Geometry: final body of the model. Coordinates: model frame, mm. A direction names the side the tool comes from. Round coordinates to 2 decimals unless told otherwise and drop trailing zeros. Loops run counter-clockwise (first coordinate to the right, second up) from the corner with the lowest first, then second, coordinate; pieces in that order, holes last. Notation, with made-up numbers: (43, 35.5) - (69, 35.5) arc R24 cw to (69, 51.5) - close; hole circle Ø8 at (-17, 15.5). An arc over 180 degrees is marked (long way). Use CSV: the item, a comma, the result in double quotes.
from build123d import *

# Parameters (mm, degrees)
BASE_FLANGE1_DEPTH = 406.4
SKETCH6_R          = 3.175
CUT_EXTRUDE1_DEPTH = 6.35
SKETCH7_R          = 3.429
CUT_EXTRUDE2_DEPTH = 6.35


# Read off the part's stored shape, not the designer's step: Base-Flange1
with BuildPart() as part:
    # Base-Flange1 outline → Base-Flange1 (new body)
    with BuildSketch(Plane(origin=(0, 0, 0), x_dir=(0, 0, -1), z_dir=(1, 0, 0))):
        with BuildLine():
            Line((0, -3.175), (38.1, -3.175))
            Line((38.1, -3.175), (38.1, 0))
            Line((38.1, 0), (0, 0))
            Line((0, 0), (0, 38.1))
            Line((0, 38.1), (-3.175, 38.1))
            Line((-3.175, 38.1), (-3.175, 0))
            ThreePointArc((-3.175, 0), (-2.24506403, -2.24506403), (0, -3.175))
        make_face()
    extrude(amount=BASE_FLANGE1_DEPTH)

    # Sketch6 → Cut-Extrude1 (cut)
    with BuildSketch(Plane.XY.offset(3.175)):
        with Locations((31.75, 19.05)):
            Circle(SKETCH6_R)
        with Locations((374.65, 19.05)):
            Circle(SKETCH6_R)
    extrude(amount=-CUT_EXTRUDE1_DEPTH, mode=Mode.SUBTRACT)

    # Sketch7 → Cut-Extrude2 (cut)
    with BuildSketch(Plane.XZ.offset(3.175)):
        with Locations(Location((25.4, -25.4, 0), (0, 0, 270))):
            Circle(SKETCH7_R)
        with Locations(Location((381, -25.4, 0), (0, 0, 270))):
            Circle(SKETCH7_R)
    extrude(amount=-CUT_EXTRUDE2_DEPTH, mode=Mode.SUBTRACT)


solid = part.part
Item 1: Material intervals for line 1 (X direction, y = -1, z = -25); line 2 (Z direction, x = 358.5, y = 36.5) (3 decimals); line 3 (Y direction, x = 279.5, z = -21.5) (3 decimals), sorted ascending.
Final values:
line 1,"x = 0 to 21.99, 28.81 to 377.59, 384.41 to 406.4"
line 2,"z = 0 to 3.175"
line 3,"y = -3.175 to 0"
Item 2: Mould query, pull axis X, two halves, no side actions, for faces 3 (the flat face through (200, 19, 0)), 4 (the flat face through (406.4, 8, 1)), 5 (the cylindrical face through (371.48, 19.19, 1.61)). Classes: released by +X, released by -X, zero draft, split by the parting line, or undercut.
Final values:
face 3,"zero draft"
face 4,"released by +X"
face 5,"undercut"
Item 3: Reachability of faces 1 (the cylindrical face through (31.06, 15.95, 1.61)), 2 (the flat face through (200, 0, -19)) from +Z, -Z, +X, -X, +Y, -Y: full face, straight path, thin tool, end or side. Return the list, or none.
Final values:
face 1,"+Z, -Z"
face 2,"-Z, +X, -X, +Y"
Item 4: Section A-A on z = -25.4. Return the cut outline in (x, y) (3 decimals).
Final values:
outline,"(0, -3.175) - (21.971, -3.175) - (21.971, 0) - (0, 0) - close; (28.829, -3.175) - (377.571, -3.175) - (377.571, 0) - (28.829, 0) - close; (384.429, -3.175) - (406.4, -3.175) - (406.4, 0) - (384.429, 0) - close"
Item 5: Section C-C on y = 27.5. Return the cut outline in (x, z) (3 decimals), plus the area to 3 significant figures.
Final values:
outline,"(0, 0) - (406.4, 0) - (406.4, 3.175) - (0, 3.175) - close"
area,"1,290 mm²"
Item 6: Section B-B on x = 133. Return the cut outline in (y, z) (3 decimals), plus the area to 3 significant figures.
Final values:
outline,"(-3.175, -38.1) - (0, -38.1) - (0, 0) - (38.1, 0) - (38.1, 3.175) - (0, 3.175) arc R3.175 ccw to (-3.175, 0) - close"
area,"250 mm²"
Item 7: Pin query (flat end, axial travel): P1, Ø19, axis at x = 189, z = -20.5, coming from the +Y side; P2, Ø2, axis at y = 1.5, z = -6, coming from the -X side. Return the tip coordinate at first contact, or that it passes through.
Final values:
P1,"stops at y = 0"
P2,"passes through"
